```python
from build123d import *

# Parameters (mm, degrees)
BOSS_EXTRUDE1_DEPTH = 5
BOSS_EXTRUDE2_DEPTH = 5
FILLET1_R           = 5
SKETCH3_R           = 5.5
SKETCH3_R_2         = 2.15
BOSS_EXTRUDE3_DEPTH = 6.75
SKETCH4_R           = 2.15
CUT_EXTRUDE1_DEPTH  = 6


with BuildPart() as part:
    # Sketch1 → Boss-Extrude1 (new body)
    with BuildSketch(Plane.XY):
        with BuildLine():
            Line((-35.355339059, 49.497474683), (-26.140144074, 40.282279698))
            Line((-26.140144074, 40.282279698), (18.49094778, 66.050052594))
            Line((18.49094778, 66.050052594), (13.651828996, 68.518195913))
            ThreePointArc((13.651828996, 68.518195913), (8.198744915, 77.166678081), (13.195371394, 86.086660909))
            Line((13.195371394, 86.086660909), (-47.426406871, 51.086660909))
            ThreePointArc((-47.426406871, 51.086660909), (-41.121144949, 52.340855485), (-35.355339059, 49.497474683))
        make_face()
        with BuildLine():
            Line((18.49094778, 66.050052594), (128.384429361, 10))
            Line((128.384429361, 10), (170, 10))
            ThreePointArc((170, 10), (172.336438573, 9.723222449), (174.543542397, 8.908210959))
            Line((174.543542397, 8.908210959), (22.738913791, 86.33461783))
            ThreePointArc((22.738913791, 86.33461783), (28.191997872, 77.686135661), (23.195371394, 68.766152833))
            Line((23.195371394, 68.766152833), (18.49094778, 66.050052594))
        make_face()
        with BuildLine():
            Line((128.384429361, 10), (4.142135624, 10))
            Line((4.142135624, 10), (7.071067812, 7.071067812))
            ThreePointArc((7.071067812, 7.071067812), (9.238795325, -3.826834324), (0, -10))
            Line((0, -10), (170, -10))
            ThreePointArc((170, -10), (167.663561427, -9.723222449), (165.456457603, -8.908210959))
            Line((165.456457603, -8.908210959), (128.384429361, 10))
        make_face()
        with BuildLine():
            ThreePointArc((-7.071067812, -7.071067812), (-9.238795325, 3.826834324), (0, 10))
            Line((0, 10), (4.142135624, 10))
            Line((4.142135624, 10), (-26.140144074, 40.282279698))
            Line((-26.140144074, 40.282279698), (-37.426406871, 33.766152833))
            ThreePointArc((-37.426406871, 33.766152833), (-43.731668793, 32.511958257), (-49.497474683, 35.355339059))
            Line((-49.497474683, 35.355339059), (-7.071067812, -7.071067812))
        make_face()
        with BuildLine():
            Line((170, 10), (128.384429361, 10))
            Line((128.384429361, 10), (165.456457603, -8.908210959))
            ThreePointArc((165.456457603, -8.908210959), (167.663561427, -9.723222449), (170, -10))
            ThreePointArc((170, -10), (179.723222449, -2.336438573), (174.543542397, 8.908210959))
            ThreePointArc((174.543542397, 8.908210959), (172.336438573, 9.723222449), (170, 10))
        make_face()
        with BuildLine():
            Line((13.651828996, 68.518195913), (18.49094778, 66.050052594))
            Line((18.49094778, 66.050052594), (23.195371394, 68.766152833))
            ThreePointArc((23.195371394, 68.766152833), (28.191997872, 77.686135661), (22.738913791, 86.33461783))
            ThreePointArc((22.738913791, 86.33461783), (17.935642604, 87.42303335), (13.195371394, 86.086660909))
            ThreePointArc((13.195371394, 86.086660909), (8.198744915, 77.166678081), (13.651828996, 68.518195913))
        make_face()
        with BuildLine():
            Line((-37.426406871, 33.766152833), (-26.140144074, 40.282279698))
            Line((-26.140144074, 40.282279698), (-35.355339059, 49.497474683))
            ThreePointArc((-35.355339059, 49.497474683), (-41.121144949, 52.340855485), (-47.426406871, 51.086660909))
            ThreePointArc((-47.426406871, 51.086660909), (-52.340855485, 43.731668793), (-49.497474683, 35.355339059))
            ThreePointArc((-49.497474683, 35.355339059), (-43.731668793, 32.511958257), (-37.426406871, 33.766152833))
        make_face()
        with BuildLine():
            Line((4.142135624, 10), (0, 10))
            ThreePointArc((0, 10), (-9.238795325, 3.826834324), (-7.071067812, -7.071067812))
            ThreePointArc((-7.071067812, -7.071067812), (-3.826834324, -9.238795325), (0, -10))
            ThreePointArc((0, -10), (9.238795325, -3.826834324), (7.071067812, 7.071067812))
            Line((7.071067812, 7.071067812), (4.142135624, 10))
        make_face()
    extrude(amount=BOSS_EXTRUDE1_DEPTH)

    # Sketch2 → Boss-Extrude2 (add, through all)
    with BuildSketch(Plane.XY.offset(5)):
        Polygon((18.49094778, 66.050052594), (10.366771374, 61.359557158), (40.019225525, 10), (57.3397336, 10), (27.687279449, 61.359557158), align=None)
    extrude(amount=-BOSS_EXTRUDE2_DEPTH)

    # Fillet1
    fillet1_edges = [part.edges().sort_by_distance(p)[0] for p in [
        (-26.140144074, 40.282279698, 2.5),
        (4.142135624, 10, 2.5),
        (128.384429361, 10, 2.5),
        (27.687279449, 61.359557158, 2.5),
        (57.3397336, 10, 2.5),
        (40.019225525, 10, 2.5),
        (10.366771374, 61.359557158, 2.5),
    ]]
    fillet(fillet1_edges, radius=FILLET1_R)

    # Sketch3 → Boss-Extrude3 (add)
    with BuildSketch(Plane.XY.offset(5)):
        with Locations((-42.426406871, 42.426406871)):
            Circle(SKETCH3_R)
        with Locations((-42.426406871, 42.426406871)):
            Circle(SKETCH3_R_2, mode=Mode.SUBTRACT)
        with Locations((1.48492424, -1.48492424)):
            Circle(SKETCH3_R)
        with Locations((1.48492424, -1.48492424)):
            Circle(SKETCH3_R_2, mode=Mode.SUBTRACT)
        with Locations((56.28492424, -1.48492424)):
            Circle(SKETCH3_R)
        with Locations((56.28492424, -1.48492424)):
            Circle(SKETCH3_R_2, mode=Mode.SUBTRACT)
        with Locations((111.08492424, -1.48492424)):
            Circle(SKETCH3_R)
        with Locations((111.08492424, -1.48492424)):
            Circle(SKETCH3_R_2, mode=Mode.SUBTRACT)
        with Locations((166.88492424, -1.48492424)):
            Circle(SKETCH3_R)
        with Locations((166.88492424, -1.48492424)):
            Circle(SKETCH3_R_2, mode=Mode.SUBTRACT)
        with Locations((10.40114276, 72.926406871)):
            Circle(SKETCH3_R)
        with Locations((10.40114276, 72.926406871)):
            Circle(SKETCH3_R_2, mode=Mode.SUBTRACT)
    extrude(amount=BOSS_EXTRUDE3_DEPTH)

    # Sketch4 → Cut-Extrude1 (cut, through all)
    with BuildSketch(Plane.XY.offset(5)):
        with Locations((-42.426406871, 42.426406871)):
            Circle(SKETCH4_R)
        with Locations((1.48492424, -1.48492424)):
            Circle(SKETCH4_R)
        with Locations((56.28492424, -1.48492424)):
            Circle(SKETCH4_R)
        with Locations((111.08492424, -1.48492424)):
            Circle(SKETCH4_R)
        with Locations((166.88492424, -1.48492424)):
            Circle(SKETCH4_R)
        with Locations((10.40114276, 72.926406871)):
            Circle(SKETCH4_R)
    extrude(amount=-CUT_EXTRUDE1_DEPTH, mode=Mode.SUBTRACT)


solid = part.part
```
Source: CAD feature listing. Evaluate the final solid. Frame: model axes, mm. A direction names the side the tool comes from. Give positions to 0.01 mm unless a question says otherwise; leave off trailing zeros. Loops run counter-clockwise (first coordinate to the right, second up) from the corner with the lowest first, then second, coordinate; pieces in that order, holes last. Notation, with made-up numbers: (7, -38) -> (53, -38) arc R36 ccw to (53, 1) -> close; hole circle Ø11 at (73, 89). An arc over 180 degrees is marked (long way). Put each result on its own line as item: value. Start each with the question number.
1) Cut plane C-C (x = 89). Return loops of the section in (y, z), then the cut area to 3 significant figures.
2) Draft query along X for faces 3 (the face through (1, -4, 11.75)), 4 (the face through (99.7, 47.08, 2.46)), 5 (the face through (9.884, 59.345, 2.465)), 6 (the face through (46.15, 29.38, 2.54)). Return one class per face: released by +X, released by -X, zero draft, split by the parting line, or undercut.
3) Cut plane A-A (z = 7). State how many separate pieces and enclosed holes the cut face has, then the cut area to 3 significant figures.
4) Material intervals for probe 1 along X at (y, z) = (-5, 11.25); probe 2 along Z at (x, y) = (35.5, 46.5); probe 3 along Y at (x, z) = (98.5, 2.5), sorted ascending.
5) Cut plane B-B (y = 25.5). Return loops of the section in (x, z), then the cut area to 3 significant figures.
6) Contact query for flat-ended pins moving along their axis: P1, Ø5, axis at x = 130, z = 2, coming from the +Y side; P2, Ø2.5, axis at x = 81, z = 2.5, coming from the +Y side; P3, Ø4, axis at x = 10.4, y = 72.93, coming from the -Z side; P4, Ø1, axis at x = 33.5, y = 10.5, coming from the +Z side. Output: stop coordinate, or through.
7) Reachability of faces 1 (the face through (35.725, 12.564, 2.465)), 2 (the face through (-16.691, 68.832, 2.465)) from +Z, -Z, +X, -X, +Y, -Y: full face, straight path, thin tool, end or side. Return the list, or none.
8) Cut plane D-D (x = -31.5). Return loops of the section in (y, z).
Results are:
1. outline: (-10, 0) -> (10, 0) -> (10, 5) -> (-10, 5) -> close; (30.09, 0) -> (52.54, 0) -> (52.54, 5) -> (30.09, 5) -> close
1. area: 212 mm2
2. face 3: zero draft
2. face 4: released by +X
2. face 5: undercut
2. face 6: undercut
3. separate pieces: 6
3. enclosed holes: 6
3. area: 483 mm2
4. probe 1: x = -2.75 to 5.72, 52.05 to 60.52, 106.85 to 115.32, 162.65 to 171.12
4. probe 2: z = 0 to 5
4. probe 3: y = -10 to 10, 25.24 to 47.69
5. outline: (-39.64, 0) -> (-11.36, 0) -> (-11.36, 5) -> (-39.64, 5) -> close; (31.07, 0) -> (48.39, 0) -> (48.39, 5) -> (31.07, 5) -> close; (97.99, 0) -> (142.01, 0) -> (142.01, 5) -> (97.99, 5) -> close
5. area: 448 mm2
6. P1: stops at y = 32.9
6. P2: stops at y = 57.26
6. P3: passes through
6. P4: stops at z = 5
7. face 1: +Z, -Z
7. face 2: +Z, -Z, -X, +Y
8. outline: (17.36, 0) -> (60.28, 0) -> (60.28, 5) -> (17.36, 5) -> close
